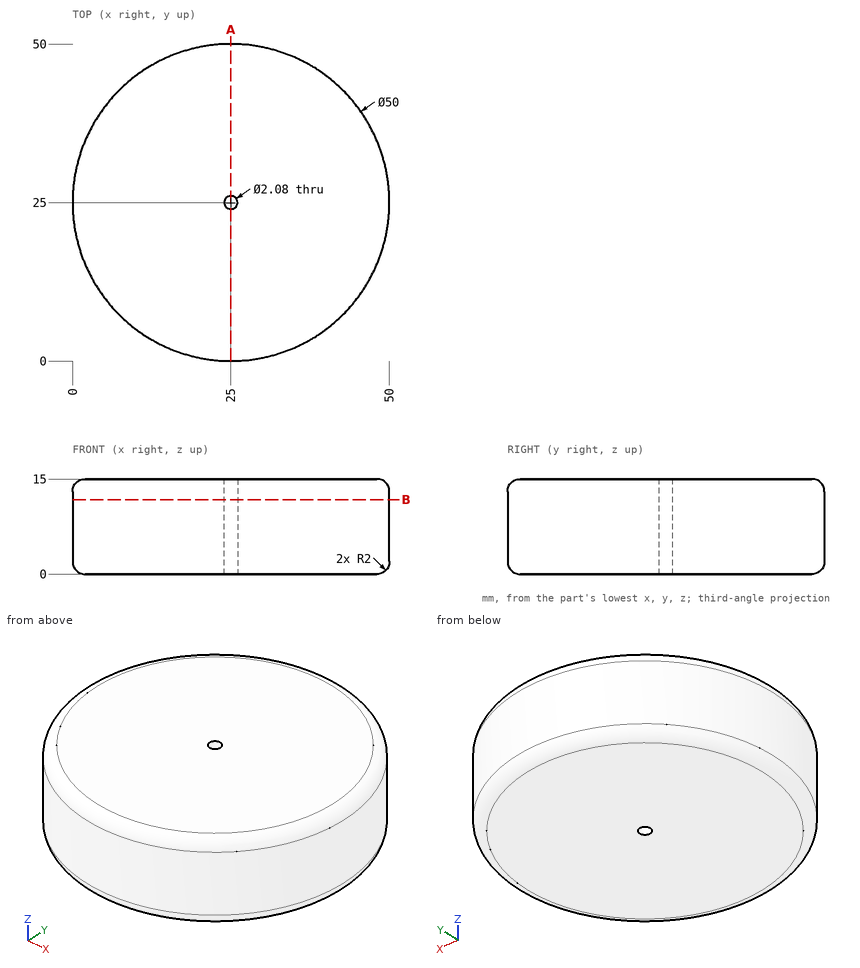
Check sheet for the drawn part. Datum: minimum x, y, z corner. Units: mm. Coordinates: 2 decimals unless noted, no trailing zeros. Loops run counter-clockwise (first coordinate to the right, second up) from the corner with the lowest first, then second, coordinate; pieces in that order, holes last. Notation, with made-up numbers: (12.5, 7) -> (19.5, 7) arc R17 cw to (19.5, 13) -> close; hole circle Ø9 at (16, -17.75). An arc over 180 degrees is marked (long way). Answer as a JSON object with one key per item and string values. Group by question number.
Item 1: Scan lines: probe 1 along Y at (x, z) = (25, 6.5); probe 2 along X at (y, z) = (24.5, 14.5); probe 3 along Z at (x, y) = (30.5, 2). Record each from-to range of solid material in increasing order.
Item 2: Sectioned sample at A-A on x = 25. Record the boundary of the cut face in (y, z).
Item 3: Depth check by flat-ended pin: pin 1 (1 mm diameter, centred on y = 14.5, z = 4, fed in from +X); pin 2 (5 mm diameter, centred on y = 39.5, z = 13, fed in from +X); pin 3 (1 mm diameter, centred on y = 5, z = 11.5, fed in from +X). Enter the tip coordinate at first touch or a pass-through.
Item 4: Sectioned sample at B-B on z = 11.75. Record the boundary of the cut face in (x, y).
Evaluation:
{
 "1": {"probe 1": "y = 0 to 23.96, 26.04 to 50", "probe 2": "x = 0.68 to 24.09, 25.91 to 49.32", "probe 3": "z = 0.11 to 14.89"},
 "2": {"outline": "(0, 2) arc R2 ccw to (2, 0) -> (23.96, 0) -> (23.96, 15) -> (2, 15) arc R2 ccw to (0, 13) -> close; (26.04, 0) -> (48, 0) arc R2 ccw to (50, 2) -> (50, 13) arc R2 ccw to (48, 15) -> (26.04, 15) -> close"},
 "3": {"pin 1": "stops at x = 47.91", "pin 2": "stops at x = 46.93", "pin 3": "stops at x = 40.64"},
 "4": {"outline": "circle Ø50 at (25, 25); hole circle Ø2.08 at (25, 25)"}
}
